CAD build for the part. Positions are in the model's coordinates, mm. A direction names the side the tool comes from. Give positions to 0.01 mm unless a question says otherwise; leave off trailing zeros. Loops run counter-clockwise (first coordinate to the right, second up) from the corner with the lowest first, then second, coordinate; pieces in that order, holes last. Notation, with made-up numbers: M 18,-18.75 L 47,-18.75 A11 ccw 47,-14.75 Z; hole C 80.5,-40 d4. An arc over 180 degrees is marked long. One line per question, with ' | ' between items.
```python
from build123d import *

# Parameters (mm, degrees)
F0_W     = 99.182904
F0_H     = 76.322906
F1_DEPTH = 38.1
F2_R     = 31.844331
F2_R_2   = 22.660652
F3_DEPTH = 25.4
F4_R     = 22.660652
F5_DEPTH = 76.2


with BuildPart() as f1:
    # F0 (on Front) → F1 (new body)
    with BuildSketch(Plane.XZ):
        Rectangle(F0_W, F0_H)
    extrude(amount=F1_DEPTH)

    # F2 (on face) → F3 (join)
    with BuildSketch(Plane.XZ.offset(38.1)):
        Circle(F2_R)
        Circle(F2_R_2, mode=Mode.SUBTRACT)
    extrude(amount=F3_DEPTH)

    # F4 (on face) → F5 (cut)
    with BuildSketch(Plane.XZ.offset(38.1)):
        Circle(F4_R)
    extrude(amount=-F5_DEPTH, mode=Mode.SUBTRACT)


solid = f1.part
```
Item 1: Drill centre lines: line 1 along Z through (x, y) = (0, -10); line 2 along Z through (x, y) = (0, -48); line 3 along Y through (x, z) = (45.5, -12). Where is each one in solid material? Low to high. Write a range as [from, to].
Conclusion:
line 1: [-38.16, -22.66], [22.66, 38.16] | line 2: [-31.84, -22.66], [22.66, 31.84] | line 3: [-38.1, 0]
Item 2: Saw through at D-D on y = -12.5. Give the cut face in (x, z).
Conclusion:
outline: M -49.59,-38.16 L 49.59,-38.16 L 49.59,38.16 L -49.59,38.16 Z; hole C 0,0 d45.32
Item 3: Saw through at B-B on x = 0. Give the cut face in (y, z).
Conclusion:
outline: M -63.5,-31.84 L -38.1,-31.84 L -38.1,-38.16 L 0,-38.16 L 0,-22.66 L -63.5,-22.66 Z; M -63.5,22.66 L 0,22.66 L 0,38.16 L -38.1,38.16 L -38.1,31.84 L -63.5,31.84 Z
Item 4: 3-axis set-ups, long thin cutter, end or side, ignore diameter. For faces 1 (the cylindrical face through (30.374, -50.622, 9.565)), 2 (the flat face through (-1, -19, 38.161)): which of +Z, -Z, +X, -X, +Y, -Y reach the whole face in a straight line?
Conclusion:
face 1: -Y | face 2: +Z, +X, -X, +Y, -Y
Item 5: Saw through at A-A on z = 0. Give the cut face in (x, y).
Conclusion:
outline: M -49.59,-38.1 L -31.84,-38.1 L -31.84,-63.5 L -22.66,-63.5 L -22.66,0 L -49.59,0 Z; M 22.66,-63.5 L 31.84,-63.5 L 31.84,-38.1 L 49.59,-38.1 L 49.59,0 L 22.66,0 Z
Item 6: Drop flat-ended pins along their axis: P1, Ø3, axis at y = -47, z = -2.5, coming from the -X side; P2, Ø10, axis at x = 31, z = -28, coming from the -Y side; P3, Ø4, axis at y = -50, z = -14.5, coming from the -X side. Give the stop position or say it passes through.
Conclusion:
P1: x = -31.83 | P2: y = -38.1 | P3: x = -29.29
Item 7: Saw through at C-C on y = -54.5. Give the cut face in (x, z).
Conclusion:
outline: C 0,0 d63.69; hole C 0,0 d45.32
